Check sheet for the modelled part. Datum: model origin and axes. Units: mm. A direction names the side the tool comes from. Coordinates: 2 decimals unless noted, no trailing zeros. Loops run counter-clockwise (first coordinate to the right, second up) from the corner with the lowest first, then second, coordinate; pieces in that order, holes last. Notation, with made-up numbers: (25.25, 85) - (57.25, 85) arc R28 ccw to (57.25, 108) - close; hole circle Ø2 at (22.25, 52.25). An arc over 180 degrees is marked (long way). Write each question's results on one line, items separated by ' | '. Start each with the question number.
1. Draft check along Z on faces 1 (the face through (5, -17, 0)), 2 (the face through (6, -26.6, -2)), 3 (the face through (12, -23, -28)). Enter one of: released by +Z, released by -Z, zero draft, split by the parting line, or undercut.
2. Gauge pin test, flat ends, axial feed: P1, Ø6, axis at x = -9.5, y = -9.5, coming from the +Z side; P2, Ø1.2, axis at x = -6, y = -13, coming from the -Z side; P3, Ø10, axis at y = -15.5, z = -19.5, coming from the +X side; P4, Ø8, axis at x = -9.5, y = -6, coming from the +Z side. Record the tip position at first contact, or that the pin passes through.
3. Cross-section at A-A (y = -23.5). Record the cut outline in (x, z), and give its area (3 significant figures).
4. Cross-section at C-C (x = 3). Record the cut outline in (y, z).
5. Thickness scan on line 1 (Y direction, x = 2.75, z = -27.75); line 2 (Z direction, x = 8, y = -9.75); line 3 (Z direction, x = 2, y = -23.5). Record the ranges inside material, lowest first. Write a range as [from, to].
6. Cross-section at B-B (z = -17.75). Record the cut outline in (x, y).
7. Tool access check on faces 4 (the face through (7, -13, -15)), 5 (the face through (6, -26, -1.3)), 6 (the face through (6, -27, -27)), 7 (the face through (-7, -15, -27)). Record the directions out of +Z, -Z, +X, -X, +Y, -Y that give a thin tool (end or side, any length) a straight path to the whole face; none if there is none.
8. Cross-section at D-D (y = -3). Record the cut outline in (x, z).
```python
from build123d import *

# Parameters (mm, degrees)
BOSS_EXTRUDE1_DEPTH = 30
SKETCH4_W           = 24
SKETCH4_H           = 14
CUT_EXTRUDE2_DEPTH  = 25
SKETCH5_W           = 1.7
SKETCH5_H           = 1.8
CUT_EXTRUDE3_DEPTH  = 15
CUT_EXTRUDE4_DEPTH  = 11
BOSS_EXTRUDE2_DEPTH = 4


with BuildPart() as part:
    # Sketch1 → Boss-Extrude1 (new body)
    with BuildSketch(Plane.XY):
        Polygon((0, 0), (0, -28), (12, -28), (12, -18), (5, 0), align=None)
    extrude(amount=-BOSS_EXTRUDE1_DEPTH)

    # Sketch4 → Cut-Extrude2 (cut)
    with BuildSketch(Plane.ZY):
        with Locations((-15, -22.638599401)):
            Rectangle(SKETCH4_W, SKETCH4_H)
    extrude(amount=-CUT_EXTRUDE2_DEPTH, mode=Mode.SUBTRACT)

    # Sketch5 → Cut-Extrude3 (cut)
    with BuildSketch(Plane.ZY):
        with Locations((-2.15, -25.7)):
            Rectangle(SKETCH5_W, SKETCH5_H)
    cut_extrude3 = extrude(amount=-CUT_EXTRUDE3_DEPTH, mode=Mode.SUBTRACT)

    # Mirror1: Cut-Extrude3 across plane
    add(cut_extrude3.mirror(Plane.XY.offset(-15)), mode=Mode.SUBTRACT)

    # Sketch6 → Cut-Extrude4 (cut, symmetric)
    with BuildSketch(Plane.XY.offset(-15)):
        Polygon((5, 0), (5, -13), (10.055555556, -13), align=None)
    extrude(amount=CUT_EXTRUDE4_DEPTH, both=True, mode=Mode.SUBTRACT)

    # Sketch7 → Boss-Extrude2 (add)
    with BuildSketch(Plane(origin=(0, -15, 0), x_dir=(1, 0, 0), z_dir=(0, 1, 0))):
        Polygon((0, 27.5), (-14.5, 27.5), (-14.5, 27), (-14.164444468, 27), (-13.881153369, 26.251032188), (-13.681153369, 26.251032188), (-13.4, 27), (-13.164444468, 27), (-12.881153369, 26.251032188), (-12.681153369, 26.251032188), (-12.4, 27), (-12.164444468, 27), (-11.881153369, 26.251032188), (-11.681153369, 26.251032188), (-11.4, 27), (-11.164444468, 27), (-10.881153369, 26.251032188), (-10.681153369, 26.251032188), (-10.4, 27), (-10.164444468, 27), (-9.881153369, 26.251032188), (-9.681153369, 26.251032188), (-9.4, 27), (-9.164444468, 27), (-8.881153369, 26.251032188), (-8.681153369, 26.251032188), (-8.4, 27), (-8.164444468, 27), (-7.881153369, 26.251032188), (-7.681153369, 26.251032188), (-7.4, 27), (-7.164444468, 27), (-6.881153369, 26.251032188), (-6.681153369, 26.251032188), (-6.4, 27), (-6.164444468, 27), (-5.881153369, 26.251032188), (-5.681153369, 26.251032188), (-5.4, 27), (-5.164444468, 27), (-4.881153369, 26.251032188), (-4.681153369, 26.251032188), (-4.4, 27), (-4.164444468, 27), (-3.881153369, 26.251032188), (-3.681153369, 26.251032188), (-3.4, 27), (-3.164444468, 27), (-2.881153369, 26.251032188), (-2.681153369, 26.251032188), (-2.4, 27), (-2.164444468, 27), (-1.881153369, 26.251032188), (-1.681153369, 26.251032188), (-1.4, 27), (-1.164444468, 27), (-0.881153369, 26.251032188), (-0.681153369, 26.251032188), (-0.4, 27), (0, 27), align=None)
    boss_extrude2 = extrude(amount=BOSS_EXTRUDE2_DEPTH)

    # Mirror2: Boss-Extrude2 across plane
    add(boss_extrude2.mirror(Plane.XY.offset(-15)))


solid = part.part
```
Established:
1) face 1: released by +Z | face 2: undercut | face 3: zero draft
2) P1: z = -2.5 | P2: z = -27.5 | P3: x = 11.08 | P4: through
3) outline: (0, -30) - (12, -30) - (12, -27) - (0, -27) - close; (0, -3) - (12, -3) - (12, 0) - (0, 0) - close | area: 72.0 mm^2
4) outline: (-28, -30) - (0, -30) - (0, 0) - (-28, 0) - (-28, -3) - (-26.6, -3) - (-26.6, -1.3) - (-24.8, -1.3) - (-24.8, -3) - (-15.64, -3) - (-15.64, -27) - (-24.8, -27) - (-24.8, -28.7) - (-26.6, -28.7) - (-26.6, -27) - (-28, -27) - close
5) line 1: [-28, -26.6], [-24.8, 0] | line 2: [-30, -26], [-4, 0] | line 3: [-30, -27], [-3, 0]
6) outline: (0, -15.64) - (11.08, -15.64) - (10.06, -13) - (5, -13) - (5, 0) - (0, 0) - close
7) face 4: +X, +Y | face 5: +X, -X | face 6: +X, -X, -Y | face 7: +Z, -Z, -X, -Y
8) outline: (0, -30) - (6.17, -30) - (6.17, -26) - (5, -26) - (5, -4) - (6.17, -4) - (6.17, 0) - (0, 0) - close
